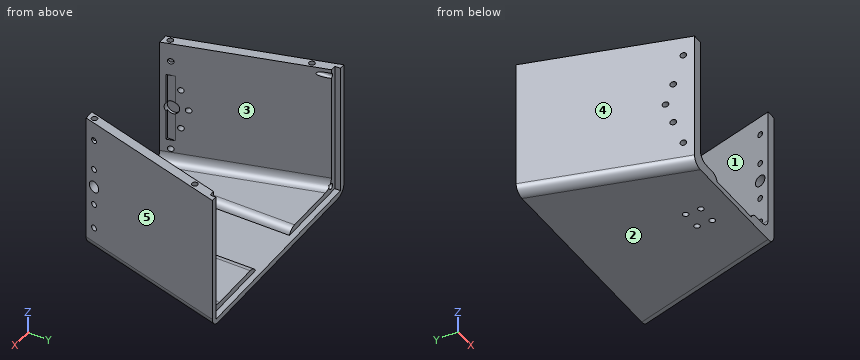
```python
from build123d import *

# Parameters (mm, degrees)
BOSS_EXTRUDE1_DEPTH     = 76
CUT_EXTRUDE1_DEPTH      = 3
CUT_EXTRUDE2_DEPTH      = 70
SKETCH4_W               = 116
SKETCH4_H               = 3
CUT_EXTRUDE3_DEPTH      = 95.00000000000003
FILLET1_R               = 5
FILLET2_R               = 5
SKETCH6_R               = 1.500000000000004
SKETCH6_R_2             = 1.4999999999999971
SKETCH6_R_3             = 1.4999999999999973
SKETCH6_R_4             = 1.5000000000000042
CUT_EXTRUDE4_DEPTH      = 10
SKETCH7_W               = 29.999999999999996
SKETCH7_H               = 5.999999999999984
CUT_EXTRUDE5_DEPTH      = 93.00000000000001
FILLET3_R               = 5
FILLET4_R               = 5
SKETCH8_R               = 1.4999999999999991
SKETCH8_R_2             = 1.5000000000000009
CUT_EXTRUDE6_DEPTH      = 93.00000000000001
SKETCH9_R               = 1.5000000000000009
SKETCH9_R_2             = 1.5000000000000042
SKETCH9_R_3             = 1.4999999999999973
CUT_EXTRUDE7_DEPTH      = 15
FILLET5_R               = 5
FILLET6_R               = 5
CUT_EXTRUDE8_DEPTH      = 30
CUT_EXTRUDE8_DEPTH_BACK = 70
SKETCH10_R              = 1.4999999999999973
SKETCH10_R_2            = 1.5000000000000009
SKETCH12_R              = 3.500000000000001
CUT_EXTRUDE9_DEPTH      = 45.6894054301587
SKETCH13_R              = 3.0000000000000018
CUT_EXTRUDE10_DEPTH     = 39.63321669991409
SKETCH15_W              = 37.000000000000014
SKETCH15_H              = 5.299999999999997
CUT_EXTRUDE13_DEPTH     = 44.38
SKETCH17_R              = 1.5000000000000042
SKETCH17_R_2            = 1.5000000000000009
CUT_EXTRUDE14_DEPTH     = 58.70047510000001
SKETCH18_R              = 1.5000000000000042
CUT_EXTRUDE15_DEPTH     = 58.70047510000001
SKETCH19_R              = 1.5000000000000042
SKETCH19_R_2            = 1.5000000000000009
CUT_EXTRUDE16_DEPTH     = 58.70047510000001


with BuildPart() as part:
    # Sketch1 → Boss-Extrude1 (new body)
    with BuildSketch(Plane.XY):
        Polygon((-70.49492385786803, 0), (45.505076142131976, 0), (22.50507614213199, -80), (-12.494923857868015, -80), (-47.494923857868024, -80), align=None)
    extrude(amount=BOSS_EXTRUDE1_DEPTH)

    # Sketch2 → Cut-Extrude1 (cut)
    with BuildSketch(Plane(origin=(0, 0, 0), x_dir=(1, 0, 0), z_dir=(0, 1, 0))):
        Polygon((-67.49492385786803, -3), (42.505076142131976, -3), (42.50507614213198, -73), (-67.49492385786802, -73), align=None)
    extrude(amount=-CUT_EXTRUDE1_DEPTH, mode=Mode.SUBTRACT)

    # Sketch3 → Cut-Extrude2 (cut)
    with BuildSketch(Plane.XY.offset(76)):
        Polygon((-42.069840297681274, -81), (17.079992581945223, -81), (39.505076142131976, -3.0000000000000124), (-64.49492385786802, -3.0000000000000124), align=None)
    extrude(amount=-CUT_EXTRUDE2_DEPTH, mode=Mode.SUBTRACT)

    # Sketch4 → Cut-Extrude3 (cut)
    with BuildSketch(Plane(origin=(0, 0, 0), x_dir=(1, 0, 0), z_dir=(0, 1, 0))):
        with Locations((-12.494923857868027, -74.5)):
            Rectangle(SKETCH4_W, SKETCH4_H)
    extrude(amount=-CUT_EXTRUDE3_DEPTH, mode=Mode.SUBTRACT)

    # Fillet1
    fillet1_edges = [part.edges().sort_by_distance(p)[0] for p in [
        (28.43628489768082, -41.50000000000001, 6),
    ]]
    fillet(fillet1_edges, radius=FILLET1_R)

    # Fillet2
    fillet2_edges = [part.edges().sort_by_distance(p)[0] for p in [
        (-53.42613261341687, -41.500000000000014, 6),
    ]]
    fillet(fillet2_edges, radius=FILLET2_R)

    # Sketch6 → Cut-Extrude4 (cut)
    with BuildSketch(Plane(origin=(0, -3, 0), x_dir=(1, 0, 0), z_dir=(0, 1, 0))):
        with Locations(Location((39.005076142131976, -6.500000000000005, 0), (0, 0, 270))):
            Circle(SKETCH6_R)
        with Locations(Location((-63.994923857868024, -6.500000000000001, 0), (0, 0, 270))):
            Circle(SKETCH6_R_2)
        with Locations(Location((-63.994923857868024, -69.49999999999999, 0), (0, 0, 270))):
            Circle(SKETCH6_R_3)
        with Locations(Location((39.00507614213195, -69.49999999999999, 0), (0, 0, 270))):
            Circle(SKETCH6_R_4)
    extrude(amount=-CUT_EXTRUDE4_DEPTH, mode=Mode.SUBTRACT)

    # Sketch7 → Cut-Extrude5 (cut)
    with BuildSketch(Plane(origin=(0, -3, 0), x_dir=(1, 0, 0), z_dir=(0, 1, 0))):
        with Locations((-12.494923857868004, -5.999999999999992)):
            Rectangle(SKETCH7_W, SKETCH7_H)
    extrude(amount=-CUT_EXTRUDE5_DEPTH, mode=Mode.SUBTRACT)

    # Fillet3
    fillet3_edges = [part.edges().sort_by_distance(p)[0] for p in [
        (34.00507614213198, -40, 0),
    ]]
    fillet(fillet3_edges, radius=FILLET3_R)

    # Fillet4
    fillet4_edges = [part.edges().sort_by_distance(p)[0] for p in [
        (-58.99492385786803, -40, 0),
    ]]
    fillet(fillet4_edges, radius=FILLET4_R)

    # Sketch8 → Cut-Extrude6 (cut)
    with BuildSketch(Plane(origin=(0, 0, 0), x_dir=(-1, 0, 0), z_dir=(0, 0, -1))):
        with Locations((7.494923857868018, -65.49999999999999)):
            Circle(SKETCH8_R)
        with Locations((7.494923857868017, -57.49999999999999)):
            Circle(SKETCH8_R_2)
        with Locations((17.494923857868017, -57.49999999999999)):
            Circle(SKETCH8_R_2)
        with Locations((17.494923857868017, -65.49999999999999)):
            Circle(SKETCH8_R_2)
    extrude(amount=-CUT_EXTRUDE6_DEPTH, mode=Mode.SUBTRACT)

    # Sketch9 → Cut-Extrude7 (cut)
    with BuildSketch(Plane.XY.offset(73)):
        with Locations((20.975017364193207, -76.5)):
            Circle(SKETCH9_R)
        with Locations((-45.964865079929254, -76.5)):
            Circle(SKETCH9_R_2)
        with Locations((-64.15615463641093, -12.999999999999998)):
            Circle(SKETCH9_R_3)
        with Locations((39.166306920674884, -13.000000000000002)):
            Circle(SKETCH9_R_2)
    extrude(amount=-CUT_EXTRUDE7_DEPTH, mode=Mode.SUBTRACT)

    # Fillet5
    # the kernel refuses this fillet: 5 mm, written as the material it takes off along each edge
    with BuildSketch(Plane(origin=(2.505076142131994, -91.45643923738959, 6), x_dir=(1, 0, 0), z_dir=(0, 1, 0))) as fillet5_piece_1:
        with BuildLine():
            CenterArc((4.582575694955839, 5), FILLET5_R, 203.57817847820183, 66.42182152179817)
            Line((-8.9e-16, 2.9999999999999996), (-0.09165151389911763, 2.9599999999999995))
            ThreePointArc((-0.09165151389911763, 2.9599999999999995), (-0.09999999999999964, 1.5), (-0.10000000000000009, 0))
            Line((-0.10000000000000009, 0), (0, -0.09999999999999964))
            Line((0, -0.09999999999999964), (4.582575694955839, -0.09999999999999964))
            Line((4.582575694955839, -0.09999999999999964), (4.582575694955839, 0))
        make_face()
    extrude(amount=99.91287847477919, mode=Mode.SUBTRACT)

    # Fillet6
    # the kernel refuses this fillet: 5 mm, written as the material it takes off along each edge
    with BuildSketch(Plane(origin=(-27.494923857868002, 8.456439237389588, 6), x_dir=(1.18e-15, 0, -1), z_dir=(0, -1, 0))) as fillet6_piece_1:
        with BuildLine():
            CenterArc((4.999999999999995, -4.582575694955842), FILLET6_R, 113.57817847820179, 66.42182152179812)
            Line((-5.43e-15, -4.582575694955835), (-0.10000000000000507, -4.582575694955835))
            Line((-0.10000000000000507, -4.582575694955835), (-0.09999999999999964, 1.2e-16))
            Line((-0.09999999999999964, 1.2e-16), (1.2e-16, 0.10000000000000142))
            ThreePointArc((1.2e-16, 0.10000000000000142), (1.4999999999999993, 0.09999999999999964), (2.959999999999998, 0.0916515138991159))
            Line((2.959999999999998, 0.0916515138991159), (2.9999999999999982, 0))
        make_face()
    extrude(amount=99.91287847477918, mode=Mode.SUBTRACT)

    # Sketch10 → Cut-Extrude8 (cut, two sides: drawn at the far end of the back side and taken through both)
    with BuildSketch(Plane(origin=(0, 0, 0), x_dir=(0, 0, -1), z_dir=(1, 0, 0)).offset(-CUT_EXTRUDE8_DEPTH_BACK)):
        with Locations(Location((-63, -75, 0), (0, 0, 90))):
            Circle(SKETCH10_R)
        with Locations(Location((-12.999999999999998, -75, 0), (0, 0, 270))):
            Circle(SKETCH10_R_2)
    extrude(amount=CUT_EXTRUDE8_DEPTH + CUT_EXTRUDE8_DEPTH_BACK, mode=Mode.SUBTRACT)

    # Sketch12 → Cut-Extrude9 (cut)
    with BuildSketch(Plane(origin=(0, 0, 0), x_dir=(0, 0, -1), z_dir=(1, 0, 0))):
        with Locations((-36.5, -74.50000000000001)):
            Circle(SKETCH12_R)
    extrude(amount=-CUT_EXTRUDE9_DEPTH, mode=Mode.SUBTRACT)

    # Sketch13 → Cut-Extrude10 (cut)
    with BuildSketch(Plane(origin=(0, 0, 0), x_dir=(0, 0, -1), z_dir=(1, 0, 0))):
        with Locations(Location((-36.5, -75.00000000000001, 0), (0, 0, 270))):
            Circle(SKETCH13_R)
    extrude(amount=CUT_EXTRUDE10_DEPTH, mode=Mode.SUBTRACT)

    # Sketch15 → Cut-Extrude13 (cut)
    with BuildSketch(Plane(origin=(0, 0, 0), x_dir=(0, 0, -1), z_dir=(1, 0, 0))):
        with Locations((-36.5, -74.5)):
            Rectangle(SKETCH15_W, SKETCH15_H)
    extrude(amount=-CUT_EXTRUDE13_DEPTH, mode=Mode.SUBTRACT)

    # Sketch17 → Cut-Extrude14 (cut)
    with BuildSketch(Plane(origin=(0, 0, 0), x_dir=(0, 0, -1), z_dir=(1, 0, 0))):
        with Locations(Location((-47.32264338558277, -70.46469184619794, 0), (0, 0, 270))):
            Circle(SKETCH17_R)
        with Locations(Location((-25.677356614417228, -70.46469184619795, 0), (0, 0, 270))):
            Circle(SKETCH17_R_2)
    extrude(amount=-CUT_EXTRUDE14_DEPTH, mode=Mode.SUBTRACT)

    # Sketch18 → Cut-Extrude15 (cut)
    with BuildSketch(Plane(origin=(0, 0, 0), x_dir=(0, 0, -1), z_dir=(1, 0, 0))):
        with Locations(Location((-36.5, -67, 0), (0, 0, 270))):
            Circle(SKETCH18_R)
    extrude(amount=-CUT_EXTRUDE15_DEPTH, mode=Mode.SUBTRACT)

    # Sketch19 → Cut-Extrude16 (cut)
    with BuildSketch(Plane(origin=(0, 0, 0), x_dir=(0, 0, -1), z_dir=(1, 0, 0))):
        with Locations(Location((-46.5, -75.00000000000001, 0), (0, 0, 270))):
            Circle(SKETCH19_R)
        with Locations(Location((-26.499999999999996, -75.00000000000001, 0), (0, 0, 270))):
            Circle(SKETCH19_R_2)
    extrude(amount=CUT_EXTRUDE16_DEPTH, mode=Mode.SUBTRACT)


solid = part.part
```
Geometry: final body of the model. Coordinates: model frame, mm. Face numbers are marked on the shaded views. A direction names the side the tool comes from. Give positions to 0.01 mm unless a question says otherwise; leave off trailing zeros. Loops run counter-clockwise (first coordinate to the right, second up) from the corner with the lowest first, then second, coordinate; pieces in that order, holes last. Notation, with made-up numbers: (-17, 10) -> (15, 10) arc R16 ccw to (15, 26) -> close; hole circle Ø4 at (16, -30.5). An arc over 180 degrees is marked (long way). Return JSON: item names as keys, results as strings.
Item 1: Pin query (flat end, axial travel): P1, Ø1.5, axis at x = -63.5, z = 7, coming from the +Y side; P2, Ø4, axis at y = -67, z = 36.5, coming from the -X side; P3, Ø4, axis at y = -75, z = 63, coming from the +X side; P4, Ø1.8, axis at x = -7.49, y = -65.5, coming from the +Z side. Return the tip coordinate at first contact, or that it passes through.
Filled in:
{"P1": "y = -13", "P2": "x = -51.81", "P3": "x = 24.52", "P4": "through"}
Item 2: Section B-B, the plane z = 63. Output: boundary loops of the cut face in (x, y), plus the area to 3 significant figures.
Filled in:
{"outline": "(-70.49, 0) -> (-49.36, -73.5) -> (-44.23, -73.5) -> (-64.49, -3) -> (-67.49, -3) -> (-67.49, 0) -> close; (-48.5, -76.5) -> (-47.49, -80) -> (-42.36, -80) -> (-43.36, -76.5) -> (-44.46, -76.5) arc R1.5 cw to (-47.46, -76.5) -> close; (17.37, -80) -> (22.51, -80) -> (23.51, -76.5) -> (22.48, -76.5) arc R1.5 cw to (19.48, -76.5) -> (18.37, -76.5) -> close; (19.24, -73.5) -> (24.37, -73.5) -> (45.51, 0) -> (42.51, 0) -> (42.51, -3) -> (39.51, -3) -> close; hole circle Ø3 at (-64.16, -13); hole circle Ø3 at (39.17, -13)", "area": "755 mm^2"}
Item 3: Access query for the marked faces 1 and 2. Directions: +Z, -Z, +X, -X, +Y, -Y. A direction counts if a zero-diameter tool reaches every point of the face in a straight line with its end or side. Return the directions, or none.
Filled in:
{"face 1": "+Z, +Y", "face 2": "-Z, +X, -X, +Y, -Y"}
Item 4: Line query: line 1 (X direction, y = -77, z = 66); line 2 (Z direction, x = 19, y = -31.5); line 3 (Z direction, x = -23, y = -70). Output: solid intervals per line, ascending.
Filled in:
{"line 1": "-48.36 to -47.38, -44.55 to -43.22, 18.23 to 19.56, 22.39 to 23.37", "line 2": "0 to 6", "line 3": "0 to 3"}
Item 5: Section A-A, the plane z = 42.5. Output: boundary loops of the cut face in (x, y).
Filled in:
{"outline": "(-70.49, 0) -> (-47.49, -80) -> (-42.36, -80) -> (-43.18, -77.15) -> (-44.38, -77.15) -> (-44.38, -72.96) -> (-64.49, -3) -> (-67.49, -3) -> (-67.49, 0) -> close; (17.37, -80) -> (22.51, -80) -> (45.51, 0) -> (42.51, 0) -> (42.51, -3) -> (39.51, -3) -> close"}
Item 6: Mould query, pull axis X, two halves, no side actions, for the marked faces 3, 4 and 5. Classes: released by +X, released by -X, zero draft, split by the parting line, or undercut.
Filled in:
{"face 3": "undercut", "face 4": "released by -X", "face 5": "released by +X"}
